Geometry check sheet. Reference: the model listing, model coordinates, mm. A direction names the side the tool comes from. Round coordinates to 2 decimals unless told otherwise and drop trailing zeros. Order: outer loops, then holes, each group sorted by start corner. A loop starts at its lowest first (then second) coordinate and runs counter-clockwise, first axis right, second up.
```python
from build123d import *

# Parameters (mm, degrees)
F1_DEPTH = 2
F2_DEPTH = 7
F3_R     = 2.99999


# Not quite as in the source:
# - a fillet or chamfer is up to 0.001 mm smaller than in the source, because OpenCascade refuses the exact size


with BuildPart() as f1:
    # F0 (on Top) → F1 (new body)
    with BuildSketch(Plane.XY):
        Polygon((10.2818826017, 7.0030450644), (-7.7181173983, 7.0030450644), (-7.7181173983, -10.9969549356), (-5.7181173983, -10.9969549356), (-5.7181173983, 5.0030450644), (10.2818826017, 5.0030450644), align=None)
        Polygon((10.2818826017, 3.0030450644), (10.2818826017, 5.0030450644), (-5.7181173983, 5.0030450644), (-5.7181173983, -10.9969549356), (-3.7181173983, -10.9969549356), (-3.7181173983, 3.0030450644), align=None)
        Polygon((10.2818826017, 1.0030450644), (10.2818826017, 3.0030450644), (-3.7181173983, 3.0030450644), (-3.7181173983, -10.9969549356), (-1.7181173983, -10.9969549356), (-1.7181173983, 1.0030450644), align=None)
        Polygon((12.2818826017, 7.0030450644), (10.2818826017, 7.0030450644), (10.2818826017, 5.0030450644), (10.2818826017, 3.0030450644), (10.2818826017, 1.0030450644), (12.2818826017, 1.0030450644), align=None)
        Polygon((-5.7181173983, -10.9969549356), (-7.7181173983, -10.9969549356), (-7.7181173983, -12.9969549356), (-1.7181173983, -12.9969549356), (-1.7181173983, -10.9969549356), (-3.7181173983, -10.9969549356), align=None)
    extrude(amount=-F1_DEPTH)

    # F0 (on Top) → F2 (join)
    with BuildSketch(Plane.XY):
        Polygon((10.2818826017, 7.0030450644), (-7.7181173983, 7.0030450644), (-7.7181173983, -10.9969549356), (-5.7181173983, -10.9969549356), (-5.7181173983, 5.0030450644), (10.2818826017, 5.0030450644), align=None)
        Polygon((10.2818826017, 1.0030450644), (10.2818826017, 3.0030450644), (-3.7181173983, 3.0030450644), (-3.7181173983, -10.9969549356), (-1.7181173983, -10.9969549356), (-1.7181173983, 1.0030450644), align=None)
        Polygon((12.2818826017, 7.0030450644), (10.2818826017, 7.0030450644), (10.2818826017, 5.0030450644), (10.2818826017, 3.0030450644), (10.2818826017, 1.0030450644), (12.2818826017, 1.0030450644), align=None)
        Polygon((-5.7181173983, -10.9969549356), (-7.7181173983, -10.9969549356), (-7.7181173983, -12.9969549356), (-1.7181173983, -12.9969549356), (-1.7181173983, -10.9969549356), (-3.7181173983, -10.9969549356), align=None)
    extrude(amount=F2_DEPTH)

    # F3 (radius 3 in the source; OpenCascade refuses exactly that, so slightly less here)
    f3_edges = [f1.edges().sort_by_distance(p)[0] for p in [
        (-1.718117, 1.003045, 2.5),
        (-7.718117, 7.003045, 2.5),
        (-7.718117, -12.996955, 2.5),
        (-1.718117, -12.996955, 2.5),
        (12.281883, 1.003045, 2.5),
        (12.281883, 7.003045, 2.5),
    ]]
    fillet(f3_edges, radius=F3_R)


solid = f1.part
```
(1) Sectioned sample at C-C, the plane y = -2.25. Record the cut outline in (x, z), and give its area (3 significant figures).
Returned:
outline: (-7.72, -2) - (-1.72, -2) - (-1.72, 7) - (-3.72, 7) - (-3.72, 0) - (-5.72, 0) - (-5.72, 7) - (-7.72, 7) - close
area: 40.0 mm2
(2) Material ranges on line 1 (Y direction, x = 7, z = 2); line 2 (X direction, y = -6.25, z = 4.25); line 3 (X direction, y = 2, z = 6.75), recorded low to high.
Returned:
line 1: y = 1 to 3, 5 to 7
line 2: x = -7.72 to -5.72, -3.72 to -1.72
line 3: x = -7.72 to -5.72, -3.72 to 11.52
(3) Sectioned sample at A-A, the plane x = 2.5. Record the cut outline in (y, z).
Returned:
outline: (1, -2) - (7, -2) - (7, 7) - (5, 7) - (5, 0) - (3, 0) - (3, 7) - (1, 7) - close
(4) Draft check along Y on faces 4 (the cylindrical face through (-2.57, -12.09, 2.56)), 5 (the flat face through (3, 3.003, 3)), 6 (the cylindrical face through (11.43, 6.1, 2.44)). Enter one of: released by +Y, released by -Y, zero draft, split by the parting line, or undercut.
Returned:
face 4: released by -Y
face 5: undercut
face 6: released by +Y
(5) Set-up check for faces 1 (the flat face through (-5.718, -3, 3)), 2 (the flat face through (2, 7.003, 2)), 3 (the flat face through (-1.718, -6, 2)): record each of +Z, -Z, +X, -X, +Y, -Y from which the full face is reachable in a straight line by a thin tool's end or side.
Returned:
face 1: +Z
face 2: +Z, -Z, +X, -X, +Y
face 3: +Z, -Z, +X, -Y
(6) Depth check by flat-ended pin: P1, Ø2, axis at y = -5.5, z = 4.5, coming from the +X side; P2, Ø6, axis at x = 5, y = 0.5, coming from the -Z side. Enter the tip coordinate at first touch or a pass-through.
Returned:
P1: stops at x = -1.72
P2: stops at z = -2
